Part model, mm, in its own coordinate system. A direction names the side the tool comes from. Round coordinates to 2 decimals unless told otherwise and drop trailing zeros. Order: outer loops, then holes, each group sorted by start corner. A loop starts at its lowest first (then second) coordinate and runs counter-clockwise, first axis right, second up. Notation, with made-up numbers: (35, -6) - (78, -6) arc R26 ccw to (78, 26) - close; hole circle Ø11 at (65, 56.25). An arc over 180 degrees is marked (long way). Answer as a JSON object with one key per item and string values.
```python
from build123d import *

# Parameters (mm, degrees)
SKETCH1_W           = 107
SKETCH1_H           = 87.7
BOSS_EXTRUDE1_DEPTH = 2.31
BOSS_EXTRUDE2_DEPTH = 10
SKETCH3_R           = 2.5
SKETCH3_R_2         = 1.2
BOSS_EXTRUDE3_DEPTH = 8
BOSS_EXTRUDE4_DEPTH = 3.85
SKETCH5_W           = 28
SKETCH5_H           = 2.7
CUT_EXTRUDE1_DEPTH  = 3.85
CUT_EXTRUDE2_DEPTH  = 107
SKETCH7_W           = 1.7
SKETCH7_H           = 11.25
BOSS_EXTRUDE5_DEPTH = 16
SKETCH8_W           = 2.5
SKETCH8_H           = 10
CUT_EXTRUDE3_DEPTH  = 102.38
BOSS_EXTRUDE6_DEPTH = 6.25
BOSS_EXTRUDE7_DEPTH = 6.25


with BuildPart() as part:
    # Sketch1 → Boss-Extrude1 (new body)
    with BuildSketch(Plane(origin=(0, 0, 0), x_dir=(1, 0, 0), z_dir=(0, 1, 0))):
        with Locations((53.5, 43.85)):
            Rectangle(SKETCH1_W, SKETCH1_H)
    extrude(amount=BOSS_EXTRUDE1_DEPTH)

    # Sketch2 → Boss-Extrude2 (add)
    with BuildSketch(Plane(origin=(0, 2.31, 0), x_dir=(1, 0, 0), z_dir=(0, 1, 0))):
        Polygon((0, 47.85), (2.466911691, 47.85), (2.466911691, 85.39), (104.846911691, 85.39), (104.846911691, 47.85), (107, 47.85), (107, 87.7), (0, 87.7), align=None)
        Polygon((0, 0), (107, 0), (107, 39.85), (104.846911691, 39.85), (104.846911691, 2.31), (2.466911691, 2.31), (2.466911691, 39.85), (0, 39.85), align=None)
    extrude(amount=BOSS_EXTRUDE2_DEPTH)

    # Sketch3 → Boss-Extrude3 (add)
    with BuildSketch(Plane(origin=(0, 2.31, 0), x_dir=(1, 0, 0), z_dir=(0, 1, 0))):
        with Locations((11.156911691, 18.85)):
            Circle(SKETCH3_R)
        with Locations((11.156911691, 18.85)):
            Circle(SKETCH3_R_2, mode=Mode.SUBTRACT)
        with Locations((96.156911691, 68.85)):
            Circle(SKETCH3_R)
        with Locations((96.156911691, 68.85)):
            Circle(SKETCH3_R_2, mode=Mode.SUBTRACT)
    extrude(amount=BOSS_EXTRUDE3_DEPTH)

    # Sketch4 → Boss-Extrude4 (add)
    with BuildSketch(Plane(origin=(0, 0, 0), x_dir=(-1, 0, 0), z_dir=(0, -1, 0))):
        Polygon((0, 0), (0, 26.416), (-4.0894, 26.416), (-4.0894, 29.1084), (-29.9974, 29.1084), (-29.9974, 24.6112), (-2.31, 24.6112), (-2.31, 2.31), (-104.69, 2.31), (-104.69, 24.6112), (-77.0026, 24.6112), (-77.0026, 29.1084), (-102.9106, 29.1084), (-102.9106, 26.416), (-107, 26.416), (-107, 0), align=None)
        Polygon((0, 62.1), (0, 87.7), (-47.32, 87.7), (-47.32, 62.1), (-9.31, 62.1), (-9.31, 64.41), (-43.3322, 64.41), (-43.3322, 85.39), (-2.31, 85.39), (-2.31, 62.1), align=None)
        Polygon((-59.68, 87.7), (-107, 87.7), (-107, 62.1), (-104.69, 62.1), (-104.69, 85.39), (-63.6678, 85.39), (-63.6678, 64.41), (-97.69, 64.41), (-97.69, 62.1), (-59.68, 62.1), align=None)
    extrude(amount=BOSS_EXTRUDE4_DEPTH)

    # Sketch5 → Cut-Extrude1 (cut)
    with BuildSketch(Plane(origin=(0, 2.31, 0), x_dir=(1, 0, 0), z_dir=(0, 1, 0))):
        with Locations((17.466911691, 27.76)):
            Rectangle(SKETCH5_W, SKETCH5_H)
        with Locations((89.846911691, 27.76)):
            Rectangle(SKETCH5_W, SKETCH5_H)
    extrude(amount=-CUT_EXTRUDE1_DEPTH, mode=Mode.SUBTRACT)

    # Sketch6 → Cut-Extrude2 (cut)
    with BuildSketch(Plane(origin=(102.9106, 0, 0), x_dir=(0, 0, -1), z_dir=(1, 0, 0))):
        Polygon((29.1084, -3.85), (26.416, -1.54), (29.1084, -1.54), align=None)
    extrude(amount=-CUT_EXTRUDE2_DEPTH, mode=Mode.SUBTRACT)

    # Sketch7 → Boss-Extrude5 (add)
    with BuildSketch(Plane(origin=(0, 2.31, 0), x_dir=(1, 0, 0), z_dir=(0, 1, 0))):
        with Locations((3.316911691, 43.855)):
            Rectangle(SKETCH7_W, SKETCH7_H)
        with Locations((103.996911691, 43.855)):
            Rectangle(SKETCH7_W, SKETCH7_H)
    extrude(amount=BOSS_EXTRUDE5_DEPTH)

    # Sketch8 → Cut-Extrude3 (cut)
    with BuildSketch(Plane(origin=(104.846911691, 0, 0), x_dir=(0, 0, -1), z_dir=(1, 0, 0))):
        with Locations((39.48, 13.31)):
            Rectangle(SKETCH8_W, SKETCH8_H)
        with Locations((48.23, 13.31)):
            Rectangle(SKETCH8_W, SKETCH8_H)
    extrude(amount=-CUT_EXTRUDE3_DEPTH, mode=Mode.SUBTRACT)

    # Sketch9 → Boss-Extrude6 (add)
    with BuildSketch(Plane.XY.offset(-40.73)):
        Polygon((104.846911691, 18.31), (106.346911691, 16.31), (104.846911691, 16.31), align=None)
    extrude(amount=-BOSS_EXTRUDE6_DEPTH)

    # Sketch10 → Boss-Extrude7 (add)
    with BuildSketch(Plane.XY.offset(-40.73)):
        Polygon((0.966911691, 16.31), (2.466911691, 16.31), (2.466911691, 18.31), align=None)
    extrude(amount=-BOSS_EXTRUDE7_DEPTH)


solid = part.part
```
Item 1: Tool access for faces 1 (the flat face through (77.003, -2, -26)), 2 (the flat face through (11, 2.31, -19)), 3 (the flat face through (105, -2, -26.416)), 4 (the flat face through (75.847, 1, -28)): list every direction of +Z, -Z, +X, -X, +Y, -Y with a clear straight run to the whole face (end or side of a thin tool).
Taken from the geometry:
{"face 1": "-Y", "face 2": "+Y", "face 3": "+X, -Y", "face 4": "+Y, -Y"}
Item 2: Probe L1, parallel to X at y = 4, z = -18.85; L2, parallel to Z at x = 68.5, y = -1.75; L3, parallel to X at y = 8.5, z = -56. List the from-to ranges inside material, lowest first. Write a range as from..to.
Taken from the geometry:
{"L1": "0..2.47, 8.66..9.96, 12.36..13.66, 104.85..107", "L2": "-87.7..-85.39, -64.41..-62.1, -2.31..0", "L3": "0..2.47, 104.85..107"}
Item 3: Two-plate mould, pull along X, no slides. Class faces 5 (the flat face through (102.911, -3, -27)), 6 (the flat face through (16, -2, -24.611)), 7 (the flat face through (104, 13, -46.98)), 8 (the flat face through (90, 1, -29.11)): pulls with the +X half, pulls with the -X half, needs draft (parallel to the pull), parting line crosses it, or undercut.
Taken from the geometry:
{"face 5": "pulls with the +X half", "face 6": "undercut", "face 7": "needs draft", "face 8": "undercut"}
Item 4: Cut at B-B (z = -68.85). Write the cut outline in (x, y), plus the area to 3 significant figures.
Taken from the geometry:
{"outline": "(0, -3.85) - (2.31, -3.85) - (2.31, 0) - (43.33, 0) - (43.33, -3.85) - (47.32, -3.85) - (47.32, 0) - (59.68, 0) - (59.68, -3.85) - (63.67, -3.85) - (63.67, 0) - (104.69, 0) - (104.69, -3.85) - (107, -3.85) - (107, 12.31) - (104.85, 12.31) - (104.85, 2.31) - (98.66, 2.31) - (98.66, 10.31) - (97.36, 10.31) - (97.36, 2.31) - (94.96, 2.31) - (94.96, 10.31) - (93.66, 10.31) - (93.66, 2.31) - (2.47, 2.31) - (2.47, 12.31) - (0, 12.31) - close", "area": "363 mm2"}
Item 5: Drop flat-ended pins along their axis: P1, Ø1.7, axis at x = 105.5, z = -44, coming from the +Y side; P2, Ø1.9, axis at y = -1.5, z = -27.5, coming from the -X side; P3, Ø2, axis at x = 96.16, z = -68.85, coming from the +Y side; P4, Ø0.8, axis at x = 3.5, z = -39, coming from the +Y side. Give the stop position or say it passes through.
Taken from the geometry:
{"P1": "y = 18.31", "P2": "x = 4.09", "P3": "y = 2.31", "P4": "y = 8.31"}
Item 6: Cut at C-C (x = 71). Write the cut outline in (y, z).
Taken from the geometry:
{"outline": "(-3.85, -87.7) - (12.31, -87.7) - (12.31, -85.39) - (2.31, -85.39) - (2.31, -2.31) - (12.31, -2.31) - (12.31, 0) - (-3.85, 0) - (-3.85, -2.31) - (0, -2.31) - (0, -62.1) - (-3.85, -62.1) - (-3.85, -64.41) - (0, -64.41) - (0, -85.39) - (-3.85, -85.39) - close"}
Item 7: Cut at D-D (z = -54). Write the cut outline in (x, y), plus the area to 3 significant figures.
Taken from the geometry:
{"outline": "(0, 0) - (107, 0) - (107, 12.31) - (104.85, 12.31) - (104.85, 2.31) - (2.47, 2.31) - (2.47, 12.31) - (0, 12.31) - close", "area": "293 mm2"}
